Geometry check sheet. Reference: the model listing, model coordinates, mm. A direction names the side the tool comes from. Coordinates: 2 decimals unless noted, no trailing zeros. Write each loop counter-clockwise with the first axis right and the second up, starting at its lowest first coordinate (ties: lowest second). Pieces come first, ordered by that corner, then holes.
Autodesk Inventor part; units mm, degrees
ref_plane "YZ Plane" through (0, 0, 0) normal (1, 0, 0) x (0, 1, 0)
ref_plane "XZ Plane" through (0, 0, 0) normal (0, 1, 0) x (-1, 0, 0)
ref_plane "XY Plane" through (0, 0, 0) normal (0, 0, 1) x (1, 0, 0)
sketch "Sketch3" plane through (0, 0, 0) normal (0, 0, 1) x (1, 0, 0)
  circle A0 centre (0, 0) radius 2
  dimension "Diameter" = 4
extrude "Extrusion1" add sketch "Sketch3" against normal blind 90
sketch "Sketch4" plane through (0, 0, 0) normal (0, 0, 1) x (1, 0, 0)
  circle A0 centre (0, 0) radius 2
  circle A1 centre (0, 0) radius 3.5
  dimension "Head_Diameter" = 7
extrude "Extrusion2" add sketch "Sketch4" along normal blind 4 contours A0 | A1
sketch "Sketch5" plane through (0, 0, 4) normal (0, 0, 1) x (1, 0, 0)
  circle A0 centre (0, 0) radius 3.5
  line L0 (1.7321, 0) -> (0.866, -1.5)
  line L1 (0.866, -1.5) -> (-0.866, -1.5)
  line L2 (-0.866, -1.5) -> (-1.7321, 0)
  line L3 (-1.7321, 0) -> (-0.866, 1.5)
  line L4 (-0.866, 1.5) -> (0.866, 1.5)
  line L5 (0.866, 1.5) -> (1.7321, 0)
  line L6 (0, 0) -> (1.7321, 0) construction
  dimension "Hex_Width" = 3
extrude "Extrusion3" cut sketch "Sketch5" against normal blind 2 contours L0 L1 L2 L3 L4 L5
thread "Thread1"
chamfer "Chamfer1" distance 0.4 angle 45 1 edges at (-3.5, 0, 4)
chamfer "Chamfer2" distance 0.2 angle 45 1 edges at (-2, 0, -90)
equation "\"d14\" = 0.5 * Chamfer"
properties part number "SCREW, SOCKET HD, P, 12.9, M4X0.7X90MM" material "Steel, MS"
1. Thickness scan on line 1 along Z through (x, y) = (1, 1.5); line 2 along Y through (x, z) = (0, -44); line 3 along Z through (x, y) = (-1.5, 0.25). Record the ranges inside material, lowest first.
Computed values:
line 1: z = -90 to 4
line 2: y = -2 to 2
line 3: z = -90 to 2
2. Sectioned sample at B-B, the plane z = -4. Record the boundary of the cut face in (x, y).
Computed values:
outline: circle Ø4 at (0, 0)
3. Draft check along Y on faces 4 (the flat face through (1.293, 0.76, 3.014)), 5 (the flat face through (0, 0, 2)), 6 (the flat face through (1.3, -1.3, 4)), 7 (the cylindrical face through (3.233, 1.341, 1.775)). Enter one of: released by +Y, released by -Y, zero draft, split by the parting line, or undercut.
Computed values:
face 4: undercut
face 5: undercut
face 6: zero draft
face 7: split by the parting line
4. Gauge pin test, flat ends, axial feed: pin 1 Ø4 at (x, y) = (0.5, 1) entering from +Z; pin 2 Ø3 at (x, z) = (1, -71) entering from -Y; pin 3 Ø4 at (y, z) = (-2.5, -61.5) entering from -X; pin 4 Ø1.5 at (x, y) = (0, 0) entering from +Z. Record the tip position at first contact, or that the pin passes through.
Computed values:
pin 1: stops at z = 4
pin 2: stops at y = -2
pin 3: stops at x = -1.94
pin 4: stops at z = 2
5. Access from +Z, -Z, +X, -X, +Y, -Y to the whole of each face (thin tool, end or side, straight path). Record for faces 1 (the flat face through (0, 0, -90)), 2 (the flat face through (0, 1.5, 3)), 3 (the cylindrical face through (0, -2, -44)).
Computed values:
face 1: -Z, +X, -X, +Y, -Y
face 2: +Z
face 3: -Z
6. Sectioned sample at A-A, the plane x = 0. Record the boundary of the cut face in (y, z).
Computed values:
outline: (-3.5, 0) - (-2, 0) - (-2, -89.8) - (-1.8, -90) - (1.8, -90) - (2, -89.8) - (2, 0) - (3.5, 0) - (3.5, 3.6) - (3.1, 4) - (1.5, 4) - (1.5, 2) - (-1.5, 2) - (-1.5, 4) - (-3.1, 4) - (-3.5, 3.6) - close
